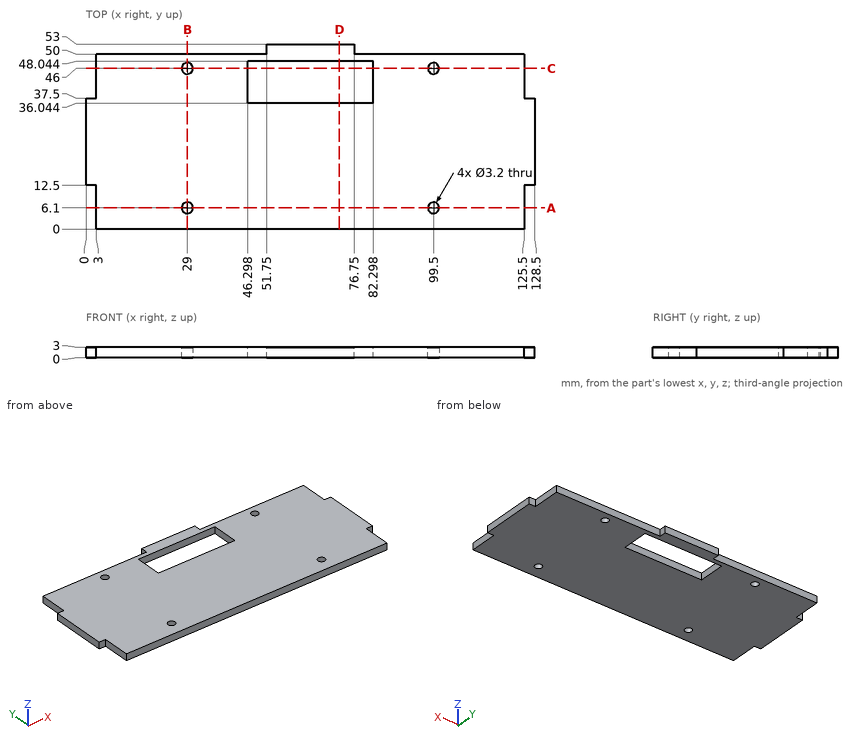
Answer from the drawing. Dimensions are ordinates in mm from the lowest x, y and z of the part. Round coordinates to 2 decimals unless told otherwise and drop trailing zeros. Order: outer loops, then holes, each group sorted by start corner. A loop starts at its lowest first (then second) coordinate and runs counter-clockwise, first axis right, second up.
1) The part is cut by section B-B on x = 29. Write down the section's boundary in (y, z), plus the area to 3 significant figures.
2) The part is cut by section A-A on y = 6.1. Write down the section's boundary in (x, z), plus the area to 3 significant figures.
3) Straight lines are drawn through the part: L1, parallel to Y at x = 99.5, z = 1.1; L2, parallel to Y at x = 68, z = 2.6; L3, parallel to Y at x = 28.5, z = 1.55. For each, find the intervals that lie inside material, in ascending order.
4) Flat-ended cylindrical pins translate along their axes: pin 1 (3.5 mm diameter, centred on x = 99.5, y = 6.1, fed in from +Z); pin 2 (0.9 mm diameter, centred on x = 127.5, z = 2, fed in from +Y); pin 3 (0.9 mm diameter, centred on x = 1.5, z = 1.5, fed in from -Y); pin 4 (1.5 mm diameter, centred on y = 8.5, z = 1, fed in from -X). Find the tip coordinate at first contact, or state that the pin passes through.
5) The part is cut by section D-D on x = 72.5. Write down the section's boundary in (y, z).
6) The part is cut by section C-C on y = 46. Write down the section's boundary in (x, z).
Resolved:
1. outline: (0, 0) - (4.5, 0) - (4.5, 3) - (0, 3) - close; (7.7, 0) - (44.4, 0) - (44.4, 3) - (7.7, 3) - close; (47.6, 0) - (50, 0) - (50, 3) - (47.6, 3) - close
1. area: 131 mm2
2. outline: (3, 0) - (27.4, 0) - (27.4, 3) - (3, 3) - close; (30.6, 0) - (97.9, 0) - (97.9, 3) - (30.6, 3) - close; (101.1, 0) - (125.5, 0) - (125.5, 3) - (101.1, 3) - close
2. area: 348 mm2
3. L1: y = 0 to 4.5, 7.7 to 44.4, 47.6 to 50
3. L2: y = 0 to 36.04, 48.04 to 53
3. L3: y = 0 to 4.58, 7.62 to 44.48, 47.52 to 50
4. pin 1: stops at z = 3
4. pin 2: stops at y = 37.5
4. pin 3: stops at y = 12.5
4. pin 4: stops at x = 3
5. outline: (0, 0) - (36.04, 0) - (36.04, 3) - (0, 3) - close; (48.04, 0) - (53, 0) - (53, 3) - (48.04, 3) - close
6. outline: (3, 0) - (27.4, 0) - (27.4, 3) - (3, 3) - close; (30.6, 0) - (46.3, 0) - (46.3, 3) - (30.6, 3) - close; (82.3, 0) - (97.9, 0) - (97.9, 3) - (82.3, 3) - close; (101.1, 0) - (125.5, 0) - (125.5, 3) - (101.1, 3) - close
